Solid Edge part; units mm, degrees
sketch "Sketch1" plane through (0, 0, 0) normal (0, 0, 1) x (1, 0, 0)
  line L0 (-98.3631, 44.16) -> (-18.3631, 44.16)
  line L1 (-18.3631, 44.16) -> (-18.3631, 104.16)
  line L2 (-18.3631, 104.16) -> (-98.3631, 104.16)
  line L3 (-98.3631, 104.16) -> (-98.3631, 44.16)
  dimension "D1" = 98.3631
  dimension "D2" = 98.3631
extrude "Protrusion1" add sketch "Sketch1" along normal blind 80
sketch "Sketch2" plane through (0, 0, 40) normal (0, 0, 1) x (1, 0, 0)
  arc A0 (-64.6899, 64.16) -> (-88.3631, 44.16) centre (-89.1875, 69.1464) cw
  line L0 (-64.6899, 64.16) -> (-64.6899, 84.16)
  arc A1 (-88.3631, 104.16) -> (-64.6899, 84.16) centre (-89.1875, 79.1736) cw
  dimension "D1" = 88.3631
  dimension "D2" = 64.6899
revolve "RevolvedCutout1" cut sketch "Sketch2" angle 360 about axis through (-58.3631, 104.16, 40) along (0, -1, 0) material side at (-73.0214, 50.0111, 40)
CAD build for the part. Positions are in the model's coordinates, mm. Give positions to 0.01 mm unless a question says otherwise; leave off trailing zeros. Write each loop counter-clockwise with the first axis right and the second up, starting at its lowest first coordinate (ties: lowest second). Pieces come first, ordered by that corner, then holes. Notation, with made-up numbers: (73.25, -2) -> (80.25, -2) arc R30 cw to (80.25, 21) -> close; hole circle Ø2 at (71.25, 63). An arc over 180 degrees is marked (long way). Return JSON: item names as keys, results as strings.
Item 1: Band-saw the part on B-B (y = 70.5). List the corners of the cut face in (x, z).
Answer below:
{"outline": "(-98.36, 0) -> (-18.36, 0) -> (-18.36, 80) -> (-98.36, 80) -> close; hole circle Ø12.65 at (-58.36, 40)"}
Item 2: Band-saw the part on A-A (z = 40). List the corners of the cut face in (x, y).
Answer below:
{"outline": "(-98.36, 44.16) -> (-88.36, 44.16) arc R25 ccw to (-64.69, 64.16) -> (-64.69, 84.16) arc R25 ccw to (-88.36, 104.16) -> (-98.36, 104.16) -> close; (-52.04, 64.16) arc R25 ccw to (-28.36, 44.16) -> (-18.36, 44.16) -> (-18.36, 104.16) -> (-28.36, 104.16) arc R25 ccw to (-52.04, 84.16) -> close"}
Item 3: Drop a flat-ended pin along its axis: pin 1 (10 mm diameter, centred on x = -58.36, z = 40, fed in from -Y). Give the stop position or say it passes through.
Answer below:
{"pin 1": "passes through"}
Item 4: Drill centre lines: probe 1 along X at (y, z) = (71, 40); probe 2 along Z at (x, y) = (-69.5, 47); probe 3 along Z at (x, y) = (-48, 51). Where is each one in solid material? Low to high.
Answer below:
{"probe 1": "x = -98.36 to -64.69, -52.04 to -18.36", "probe 2": "z = 0 to 24.33, 55.67 to 80", "probe 3": "z = 0 to 31.15, 48.85 to 80"}
Item 5: Two-plate mould, pull along Z, no slides. Class faces 1 (the flat face through (-98.363, 75, 39)), 2 (the flat face through (-59, 75, 80)), 3 (the cylindrical face through (-64.398, 74.3, 41.9)): +Z half, -Z half, draft (parallel to the pull), parting line (faces both ways), or undercut.
Answer below:
{"face 1": "draft", "face 2": "+Z half", "face 3": "undercut"}
Item 6: Band-saw the part on C-C (y = 98). List the corners of the cut face in (x, z).
Answer below:
{"outline": "(-98.36, 0) -> (-18.36, 0) -> (-18.36, 80) -> (-98.36, 80) -> close; hole circle Ø28.75 at (-58.36, 40)"}
